```python
from build123d import *

# Parameters (mm, degrees)
CHANFREIN1_SIZE              = 1.195722403
CHANFREIN1_SIZE2             = 1
CHANFREIN1_EDGE_2_SIZE       = 1.247139839
CHANFREIN1_EDGE_2_SIZE2      = 1
ENL_V_MAT_EXTRU_1_DEPTH      = 17
ENL_V_MAT_EXTRU_1_DEPTH_BACK = 17


with BuildPart() as part:
    # Esquisse1 → Révolution1 (revolve)
    with BuildSketch(Plane.XY, mode=Mode.PRIVATE) as r_volution1_sk:
        Polygon((-127.5, 0), (-127.5, 9), (-112.5, 9), (-112.5, 11), (-80, 16), (80, 16), (112.5, 10), (112.5, 8), (127.5, 8), (127.5, 0), align=None)
    revolve(r_volution1_sk.sketch.rotate(Axis((-127.5, 0, 0), (1, 0, 0)), 90), axis=Axis((-127.5, 0, 0), (1, 0, 0)))  # turned: the seam where the file's is

    # Chanfrein1
    chanfrein1_edges = [part.edges().sort_by_distance(p)[0] for p in [
        (-112.5, 0, -11),
    ]]
    chanfrein1_side = [part.faces().sort_by_distance(p)[0] for p in [
        (-112.5, 0, -9.311126984),
    ]]
    chamfer(chanfrein1_edges, length=CHANFREIN1_SIZE, length2=CHANFREIN1_SIZE2, reference=chanfrein1_side[0])

    # Chanfrein1 edge 2
    chanfrein1_edge_2_edges = [part.edges().sort_by_distance(p)[0] for p in [
        (112.5, 0, -10),
    ]]
    chanfrein1_edge_2_side = [part.faces().sort_by_distance(p)[0] for p in [
        (96.25, 0, -13),
    ]]
    chamfer(chanfrein1_edge_2_edges, length=CHANFREIN1_EDGE_2_SIZE, length2=CHANFREIN1_EDGE_2_SIZE2, reference=chanfrein1_edge_2_side[0])

    # Esquisse2 → Enlèv. mat.-Extru.1 (cut, two sides)
    with BuildSketch(Plane(origin=(0, 0, 0), x_dir=(1, 0, 0), z_dir=(0, 1, 0))) as enl_v_mat_extru_1_sk:
        Polygon((-25, 16), (-24.322079679, 11.176346273), (10, 16), align=None)
    extrude(amount=ENL_V_MAT_EXTRU_1_DEPTH, mode=Mode.SUBTRACT)
    extrude(enl_v_mat_extru_1_sk.sketch, amount=-ENL_V_MAT_EXTRU_1_DEPTH_BACK, mode=Mode.SUBTRACT)


solid = part.part
```
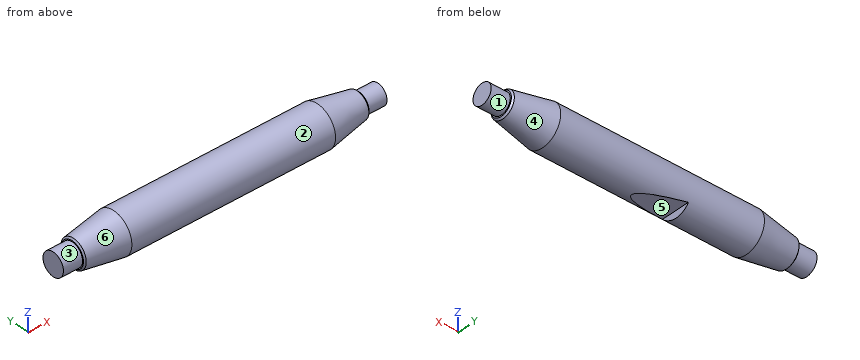
Read the model definition and answer for the solid it produces. Units are mm, in the model's axes. Face numbers are marked on the shaded views. A direction names the side the tool comes from. Give positions to 0.01 mm unless a question says otherwise; leave off trailing zeros. Order: outer loops, then holes, each group sorted by start corner. A loop starts at its lowest first (then second) coordinate and runs counter-clockwise, first axis right, second up.
(1) Given pin 1 (4 mm diameter, centred on x = 75.5, z = 2.5, fed in from -Y); pin 2 (3 mm diameter, centred on x = -17, y = -3, fed in from -Z); pin 3 (3 mm diameter, centred on x = 71.5, y = -8.5, fed in from -Z), each flat-ended and moving along its own axis, determine where each tip first touches the part or whether it passes through.
(2) Find section D-D (x = 7). Give the vertices of the cut face in (y, z), plus the area to 3 significant figures.
(3) For a pull along X with two mould halves and no side action, classify the marked faces 4, 5 and 6 as released by +X, released by -X, zero draft, split by the parting line, or undercut.
(4) For the marked faces 1, 2 and 3, determine the directions among +Z, -Z, +X, -X, +Y, -Y from which every point of the face is accessible in a straight line to the end or side of a thin tool.
(5) Find section A-A (z = 0). Give the vertices of the cut face in (x, y).
(6) Straight lines are drawn through the part: L1, parallel to X at y = 5.5, z = 6; L2, parallel to Z at x = -32, y = -0.5; L3, parallel to Y at x = -105.5, z = -3.5. For each, find the intervals that lie inside material, in ascending order.
(7) Find section B-B (y = 0). Give the vertices of the cut face in (x, z), plus the area to 3 significant figures.
(8) Find section C-C (x = -100). Give the vertices of the cut face in (y, z), plus the area to 3 significant figures.
Result sheet:
1. pin 1: stops at y = -15.99
1. pin 2: stops at z = -12.42
1. pin 3: stops at z = -14.39
2. outline: (-3.65, -15.58) - (3.65, -15.58) arc R16 ccw (long way) to start
2. area: 802 mm2
3. face 4: released by +X
3. face 5: undercut
3. face 6: released by -X
4. face 1: +X
4. face 2: +X, -X
4. face 3: -X
5. outline: (-127.5, -9) - (-112.5, -9) - (-112.5, -9.8) - (-111.51, -11.15) - (-80, -16) - (80, -16) - (111.27, -10.23) - (112.5, -9) - (112.5, -8) - (127.5, -8) - (127.5, 8) - (112.5, 8) - (112.5, 9) - (111.27, 10.23) - (80, 16) - (-80, 16) - (-111.51, 11.15) - (-112.5, 9.8) - (-112.5, 9) - (-127.5, 9) - close
6. L1: x = -127.5 to 112.5
6. L2: z = -15.99 to 15.99
6. L3: y = -11.56 to 11.56
7. outline: (-127.5, -9) - (-112.5, -9) - (-112.5, -9.8) - (-111.51, -11.15) - (-80, -16) - (-25, -16) - (-24.32, -11.18) - (10, -16) - (80, -16) - (111.27, -10.23) - (112.5, -9) - (112.5, -8) - (127.5, -8) - (127.5, 8) - (112.5, 8) - (112.5, 9) - (111.27, 10.23) - (80, 16) - (-80, 16) - (-111.51, 11.15) - (-112.5, 9.8) - (-112.5, 9) - (-127.5, 9) - close
7. area: 7,270 mm2
8. outline: circle Ø25.85 at (0, 0)
8. area: 525 mm2
